Work out the finished part from the listing and answer in its coordinate system (mm). Face numbers are marked on the shaded views. Give positions to 0.01 mm unless a question says otherwise; leave off trailing zeros. Write each loop counter-clockwise with the first axis right and the second up, starting at its lowest first coordinate (ties: lowest second). Pieces come first, ordered by that corner, then holes. Notation, with made-up numbers: (-1.75, 33.5) -> (43.25, 33.5) arc R10 ccw to (43.25, 51.5) -> close; hole circle Ø7 at (0, -9.75). An arc over 180 degrees is marked (long way). Write item = value, one per line. Start each with the question number.
from build123d import *

# Parameters (mm, degrees)
SKETCH_1_R      = 1.5
SKETCH_1_R_2    = 10.875
EXTRUDE_1_DEPTH = 3


with BuildPart() as part:
    # Эскиз1 → Бобышка-Вытянуть1 (new body)
    with BuildSketch(Plane.XY):
        Polygon((17.25, 21), (21, 17.25), (21, -17.25), (17.25, -21), (-17.25, -21), (-21, -17.25), (-21, 17.25), (-17.25, 21), align=None)
        with Locations((-15.5, 15.5)):
            Circle(SKETCH_1_R, mode=Mode.SUBTRACT)
        with Locations((15.5, 15.5)):
            Circle(SKETCH_1_R, mode=Mode.SUBTRACT)
        with Locations((15.5, -15.5)):
            Circle(SKETCH_1_R, mode=Mode.SUBTRACT)
        with Locations((-15.5, -15.5)):
            Circle(SKETCH_1_R, mode=Mode.SUBTRACT)
        Circle(SKETCH_1_R_2, mode=Mode.SUBTRACT)
    extrude(amount=EXTRUDE_1_DEPTH)


solid = part.part
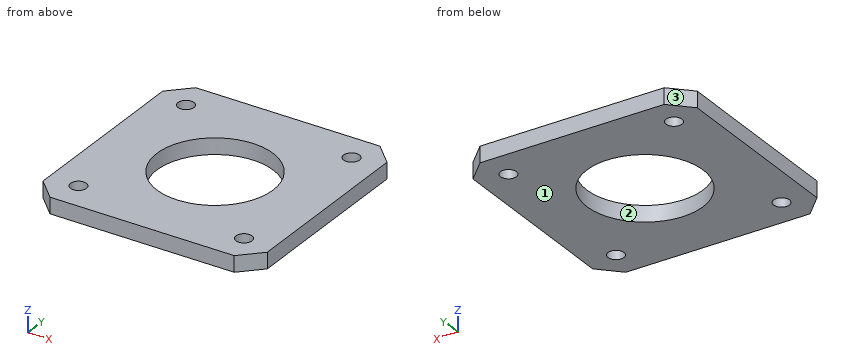
(1) Determine the mould class of the marked faces 1, 2 and 3 for opening direction X: pulls with the +X half, pulls with the -X half, needs draft (parallel to the pull), parting line crosses it, or undercut.
(2) A cutting plane is placed at D-D, the plane z = 1.45. Write down the section's boundary in (x, y) (3 decimals).
(3) Find the intervals of material crossed by line 1 along Y through (x, z) = (-15.5, 1.75); line 2 along X through (y, z) = (16.5, 1.15); line 3 along Y through (x, z) = (15, 0.8), in increasing order.
(4) A cutting plane is placed at B-B, the plane x = 15.5. Write down the section's boundary in (y, z).
(5) A cutting plane is placed at A-A, the plane y = 0. Write down the section's boundary in (x, z) (3 decimals), then the cut area to 4 significant figures.
Results list:
q1.face_1 = needs draft
q1.face_2 = undercut
q1.face_3 = pulls with the -X half
q2.outline = (-21, -17.25) -> (-17.25, -21) -> (17.25, -21) -> (21, -17.25) -> (21, 17.25) -> (17.25, 21) -> (-17.25, 21) -> (-21, 17.25) -> close; hole circle Ø3 at (-15.5, -15.5); hole circle Ø3 at (-15.5, 15.5); hole circle Ø21.75 at (0, 0); hole circle Ø3 at (15.5, -15.5); hole circle Ø3 at (15.5, 15.5)
q3.line_1 = -21 to -17, -14 to 14, 17 to 21
q3.line_2 = -21 to -16.62, -14.38 to 14.38, 16.62 to 21
q3.line_3 = -21 to -16.91, -14.09 to 14.09, 16.91 to 21
q4.outline = (-21, 0) -> (-17, 0) -> (-17, 3) -> (-21, 3) -> close; (-14, 0) -> (14, 0) -> (14, 3) -> (-14, 3) -> close; (17, 0) -> (21, 0) -> (21, 3) -> (17, 3) -> close
q5.outline = (-21, 0) -> (-10.875, 0) -> (-10.875, 3) -> (-21, 3) -> close; (10.875, 0) -> (21, 0) -> (21, 3) -> (10.875, 3) -> close
q5.area = 60.75 mm²
